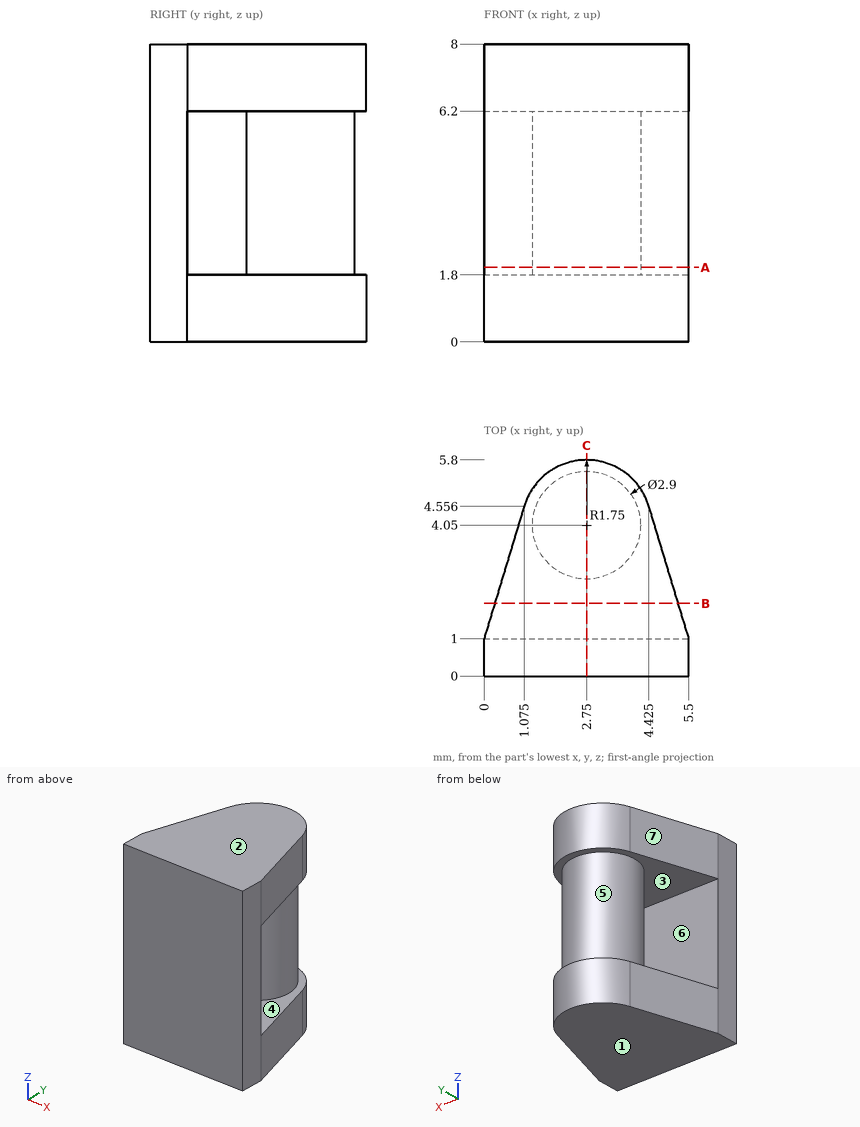
For this review, use the dimensioned drawing (mm, ordinates from the lowest corner) and the shaded views. A direction names the side the tool comes from. Give positions to 0.01 mm unless a question says otherwise; leave off trailing zeros. Write each loop counter-clockwise with the first axis right and the second up, starting at its lowest first coordinate (ties: lowest second). Pieces come first, ordered by that corner, then holes. Notation, with made-up numbers: M -25,-4.5 L 13,-4.5 A18 ccw 13,25.5 Z; hole C 10.5,83 d9. An arc over 180 degrees is marked long. Answer as a JSON object with one key per item and string values. Group by question number.
Item 1: Draft analysis for pull direction Z (two halves, no side actions). For the marked faces 1, 2, 3 and 4, state which applies: +Z half, -Z half, draft (parallel to the pull), parting line (faces both ways), or undercut.
Item 2: Consider section B-B on y = 1.95. Write out the cut boundary in (x, z).
Item 3: For pin 1 Ø1 at (x, y) = (3, 1) entering from -Z; pin 2 Ø1.3 at (x, z) = (2, 4) entering from +Y, all flat-tipped, find the tip position at first contact; note any pin that passes through.
Item 4: For probe 1 along Z at (x, y) = (4.45, 3.55); probe 2 along Y at (x, z) = (2.85, 7.25); probe 3 along Y at (x, z) = (0.45, 4), list the stretches that pass through material, from the lowest coordinate up. Write a range as [from, to].
Item 5: Consider section C-C on x = 2.75. Write out the cut boundary in (y, z).
Item 6: Consider section A-A on z = 2. Write out the cut boundary in (x, y), plus the area to 3 significant figures.
Item 7: Tool access review of the marked faces 5, 6 and 7: name each direction out of +Z, -Z, +X, -X, +Y, -Y from which nothing blocks a thin tool from reaching the whole face with its end or side.
Check result:
{
 "1": {"face 1": "-Z half", "face 2": "+Z half", "face 3": "undercut", "face 4": "undercut"},
 "2": {"outline": "M 0.29,0 L 5.21,0 L 5.21,1.8 L 0.29,1.8 Z; M 0.29,6.2 L 5.21,6.2 L 5.21,8 L 0.29,8 Z"},
 "3": {"pin 1": "stops at z = 0", "pin 2": "stops at y = 5.5"},
 "4": {"probe 1": "z = [0, 1.8], [6.2, 8]", "probe 2": "y = [0, 5.8]", "probe 3": "y = [0, 1]"},
 "5": {"outline": "M 0,0 L 5.8,0 L 5.8,1.8 L 5.5,1.8 L 5.5,6.2 L 5.8,6.2 L 5.8,8 L 0,8 Z; hole M 1,1.8 L 2.6,1.8 L 2.6,6.2 L 1,6.2 Z"},
 "6": {"outline": "M 0,0 L 5.5,0 L 5.5,1 L 0,1 Z; C 2.75,4.05 d2.9", "area": "12.1 mm^2"},
 "7": {"face 5": "none", "face 6": "+X, -X", "face 7": "+Z, -Z, -X, +Y"}
}
